```python
from build123d import *

# Parameters (mm, degrees)
BOSS_EXTRUDE1_DEPTH = 184.15
SKETCH2_R           = 1.651
SKETCH2_R_2         = 2.0701
SKETCH2_R_3         = 2.0955
CUT_EXTRUDE3_DEPTH  = 10


with BuildPart() as part:
    # Sketch1 → Boss-Extrude1 (new body)
    with BuildSketch(Plane.XY):
        Polygon((0, 26.6954), (0, 4.7498), (0, 0), (61.849, 0), (69.342, 0), (90.932, 0), (90.932, 4.7498), (69.342, 4.7498), (61.849, 4.7498), (61.849, 26.6954), (59.436, 26.6954), (59.436, 4.7498), (51.943, 4.7498), (51.943, 26.6954), (49.53, 26.6954), (49.53, 4.7498), (42.037, 4.7498), (42.037, 26.6954), (39.624, 26.6954), (39.624, 4.7498), (32.131, 4.7498), (32.131, 26.6954), (29.718, 26.6954), (29.718, 4.7498), (22.225, 4.7498), (22.225, 26.6954), (19.812, 26.6954), (19.812, 4.7498), (12.319, 4.7498), (12.319, 26.6954), (9.906, 26.6954), (9.906, 4.7498), (2.413, 4.7498), (2.413, 26.6954), align=None)
    extrude(amount=BOSS_EXTRUDE1_DEPTH)

    # Sketch2 → Cut-Extrude3 (cut)
    with BuildSketch(Plane.XZ):
        with Locations((5.2324, 159.131)):
            Circle(SKETCH2_R)
        with Locations((44.8056, 180.467)):
            Circle(SKETCH2_R)
        with Locations((44.8056, 143.243)):
            Circle(SKETCH2_R)
        with Locations((5.2324, 121.907)):
            Circle(SKETCH2_R)
        with Locations((5.2324, 84.683)):
            Circle(SKETCH2_R)
        with Locations((44.8056, 106.019)):
            Circle(SKETCH2_R)
        with Locations((17.0185, 72.3)):
            Circle(SKETCH2_R_2)
        with Locations((25.0185, 72.3)):
            Circle(SKETCH2_R_2)
        with Locations((25.0185, 5.7)):
            Circle(SKETCH2_R_2)
        with Locations((17.0185, 5.7)):
            Circle(SKETCH2_R_2)
        with Locations((38.317522863, 39)):
            Circle(SKETCH2_R_3)
    extrude(amount=-CUT_EXTRUDE3_DEPTH, mode=Mode.SUBTRACT)


solid = part.part
```
Model file for the job. Use its own axes, mm. A direction names the side the tool comes from. Coordinates: 2 decimals unless noted, no trailing zeros. Loops run counter-clockwise (first coordinate to the right, second up) from the corner with the lowest first, then second, coordinate; pieces in that order, holes last. Notation, with made-up numbers: (61.25, 88.25) - (76.25, 88.25) arc R23 cw to (76.25, 96.25) - close; hole circle Ø3 at (72, 36.25). An arc over 180 degrees is marked (long way). Answer as a JSON object with one key per item and string values. Group by question number.
(1) Tool access for faces 3 (the face through (22.225, 16, 91)), 4 (the face through (31.8, 9.5, 184.15)), 5 (the face through (40.316, 2.708, 39.629)): list every direction of +Z, -Z, +X, -X, +Y, -Y with a clear straight run to the whole face (end or side of a thin tool).
(2) Probe line 1 along Y through (x, z) = (77.5, 74). List the from-to ranges inside material, lowest first.
(3) Cut at A-A (y = 7.5). State how many separate pieces and enclosed holes the cut face has, then the cut area to 3 significant figures.
(4) Flat gauge pins, fed straight in: pin 1 (4 mm diameter, centred on x = 44.81, z = 180.47, fed in from +Y); pin 2 (8 mm diameter, centred on y = 12.5, z = 19, fed in from +X). Where does each tip first touch, or does it go through?
(5) Two-plate mould, pull along X, no slides. Class faces 1 (the face through (12.319, 16, 91)), 2 (the face through (77, 4.75, 91)): released by +X, released by -X, zero draft, split by the parting line, or undercut.
(6) Cut at C-C (y = 15.5). Give the cut face in (x, z) (3 decimals).
Geometry says:
{
 "1": {"face 3": "+Z, -Z, +Y", "face 4": "+Z, +X, -X, +Y, -Y", "face 5": "-Y"},
 "2": {"line 1": "y = 0 to 4.75"},
 "3": {"separate pieces": "7", "enclosed holes": "0", "area": "3,110 mm^2"},
 "4": {"pin 1": "stops at y = 4.75", "pin 2": "stops at x = 61.85"},
 "5": {"face 1": "undercut", "face 2": "zero draft"},
 "6": {"outline": "(0, 0) - (2.413, 0) - (2.413, 184.15) - (0, 184.15) - close; (9.906, 0) - (12.319, 0) - (12.319, 184.15) - (9.906, 184.15) - close; (19.812, 0) - (22.225, 0) - (22.225, 184.15) - (19.812, 184.15) - close; (29.718, 0) - (32.131, 0) - (32.131, 184.15) - (29.718, 184.15) - close; (39.624, 0) - (42.037, 0) - (42.037, 184.15) - (39.624, 184.15) - close; (49.53, 0) - (51.943, 0) - (51.943, 184.15) - (49.53, 184.15) - close; (59.436, 0) - (61.849, 0) - (61.849, 184.15) - (59.436, 184.15) - close"}
}
